CAD build for the part. Positions are in the model's coordinates, mm. Round coordinates to 2 decimals unless told otherwise and drop trailing zeros. Write each loop counter-clockwise with the first axis right and the second up, starting at its lowest first coordinate (ties: lowest second). Pieces come first, ordered by that corner, then holes. Notation, with made-up numbers: (34, 39.25) - (91, 39.25) arc R31 ccw to (91, 63.25) - close; hole circle Ø9 at (33.5, 16.25). An arc over 180 degrees is marked (long way). Answer in a Markdown table with one row per item.
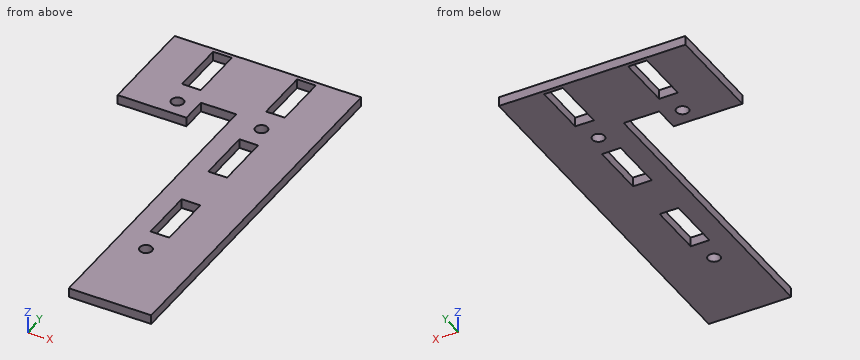
```python
from build123d import *

# Parameters (mm, degrees)
SKETCH1_W           = 101.6
SKETCH1_H           = 50.8
BOSS_EXTRUDE1_DEPTH = 2.54
SKETCH2_R           = 1.651
CUT_EXTRUDE1_DEPTH  = 57.852894385
SKETCH3_W           = 5.1
SKETCH3_H           = 15.02
CUT_EXTRUDE4_DEPTH  = 57.852894385
CUT_EXTRUDE5_DEPTH  = 57.852894385


with BuildPart() as part:
    # Sketch1 → Boss-Extrude1 (new body)
    with BuildSketch(Plane(origin=(0, 0, 0), x_dir=(0, 1, 0), z_dir=(0, 0, 1))):
        Rectangle(SKETCH1_W, SKETCH1_H)
    extrude(amount=BOSS_EXTRUDE1_DEPTH)

    # Sketch2 → Cut-Extrude1 (cut, through all)
    with BuildSketch(Plane.XY.offset(2.54)):
        with Locations((11.115903034, 27.94)):
            Circle(SKETCH2_R)
        with Locations((11.115903034, -27.94)):
            Circle(SKETCH2_R)
        with Locations((-11.744096966, 27.94)):
            Circle(SKETCH2_R)
    extrude(amount=-CUT_EXTRUDE1_DEPTH, mode=Mode.SUBTRACT)

    # Sketch3 → Cut-Extrude4 (cut, through all)
    with BuildSketch(Plane.XY.offset(2.54)):
        with Locations((11.115903034, -13.67)):
            Rectangle(SKETCH3_W, SKETCH3_H)
        with Locations((11.115903034, 14.27)):
            Rectangle(SKETCH3_W, SKETCH3_H)
        with Locations((11.115903034, 42.21)):
            Rectangle(SKETCH3_W, SKETCH3_H)
        with Locations((-11.744096966, 42.21)):
            Rectangle(SKETCH3_W, SKETCH3_H)
    extrude(amount=-CUT_EXTRUDE4_DEPTH, mode=Mode.SUBTRACT)

    # Sketch5 → Cut-Extrude5 (cut, through all)
    with BuildSketch(Plane.XY.offset(2.54)):
        Polygon((2.977903034, -50.8), (2.977903034, 30.255), (-6.674096966, 30.255), (-6.674096966, 23.27), (-25.4, 23.27), (-25.4, -50.8), align=None)
    extrude(amount=-CUT_EXTRUDE5_DEPTH, mode=Mode.SUBTRACT)


solid = part.part
```
Q1. Drill centre lines: line 1 (X direction, y = 35.5, z = 0.2); line 2 (Y direction, x = 11, z = 0.7); line 3 (X direction, y = -6.5, z = 1.2). Where is each one in solid material? Low to high.
Computed:
| item | result |
|---|---|
| line 1 | x = -25.4 to -14.29, -9.19 to 8.57, 13.67 to 25.4 |
| line 2 | y = -50.8 to -29.59, -26.29 to -21.18, -6.16 to 6.76, 21.78 to 26.29, 29.59 to 34.7, 49.72 to 50.8 |
| line 3 | x = 2.98 to 8.57, 13.67 to 25.4 |
Q2. Saw through at C-C on y = 12. List the corners of the cut face in (x, z), then the cut area to 3 significant figures.
Computed:
| item | result |
|---|---|
| outline | (2.98, 0) - (8.57, 0) - (8.57, 2.54) - (2.98, 2.54) - close; (13.67, 0) - (25.4, 0) - (25.4, 2.54) - (13.67, 2.54) - close |
| area | 44.0 mm2 |
Q3. Saw through at A-A on y = 43.5. List the corners of the cut face in (x, z), then the cut area to 3 significant figures.
Computed:
| item | result |
|---|---|
| outline | (-25.4, 0) - (-14.29, 0) - (-14.29, 2.54) - (-25.4, 2.54) - close; (-9.19, 0) - (8.57, 0) - (8.57, 2.54) - (-9.19, 2.54) - close; (13.67, 0) - (25.4, 0) - (25.4, 2.54) - (13.67, 2.54) - close |
| area | 103 mm2 |
Q4. Saw through at D-D on y = 27.94. List the corners of the cut face in (x, z).
Computed:
| item | result |
|---|---|
| outline | (-25.4, 0) - (-13.4, 0) - (-13.4, 2.54) - (-25.4, 2.54) - close; (-10.09, 0) - (-6.67, 0) - (-6.67, 2.54) - (-10.09, 2.54) - close; (2.98, 0) - (9.46, 0) - (9.46, 2.54) - (2.98, 2.54) - close; (12.77, 0) - (25.4, 0) - (25.4, 2.54) - (12.77, 2.54) - close |
Q5. Saw through at B-B on z = 1.6. List the corners of the cut face in (x, y) (3 decimals).
Computed:
| item | result |
|---|---|
| outline | (-25.4, 23.27) - (-6.674, 23.27) - (-6.674, 30.255) - (2.978, 30.255) - (2.978, -50.8) - (25.4, -50.8) - (25.4, 50.8) - (-25.4, 50.8) - close; hole (-14.294, 34.7) - (-9.194, 34.7) - (-9.194, 49.72) - (-14.294, 49.72) - close; hole circle Ø3.302 at (-11.744, 27.94); hole (8.566, -21.18) - (13.666, -21.18) - (13.666, -6.16) - (8.566, -6.16) - close; hole (8.566, 6.76) - (13.666, 6.76) - (13.666, 21.78) - (8.566, 21.78) - close; hole (8.566, 34.7) - (13.666, 34.7) - (13.666, 49.72) - (8.566, 49.72) - close; hole circle Ø3.302 at (11.116, -27.94); hole circle Ø3.302 at (11.116, 27.94) |
Q6. Flat gauge pins, fed straight in: pin 1 (0.8 mm diameter, centred on y = -13.5, z = 2, fed in from -X); pin 2 (1.3 mm diameter, centred on x = -19, z = 1, fed in from -Y). Where does each tip first touch, or does it go through?
Computed:
| item | result |
|---|---|
| pin 1 | stops at x = 2.98 |
| pin 2 | stops at y = 23.27 |
